from build123d import *

# Parameters (mm, degrees)
F0_R          = 10
F1_DEPTH      = 45
F1_DEPTH_BACK = 95
F0_R_2        = 15
F2_DEPTH      = 65
F4_START      = 7.5
F4_DEPTH      = 17.5
F6_DEPTH      = 30
F7_R          = 2
F8_DEPTH      = 25
F9_R          = 2
F10_DEPTH     = 25
F11_R         = 2
F12_DEPTH     = 25
F13_R         = 2
F14_DEPTH     = 25
F16_D         = 5
F16_DEPTH     = 20
F16_TIP       = 1.5021515476
F17_R         = 11.65
F18_DEPTH     = 1


with BuildPart() as f1:
    # F0 (on Front) → F1 (new body, two sides)
    with BuildSketch(Plane.XZ) as f1_sk:
        Circle(F0_R)
    extrude(amount=F1_DEPTH)
    extrude(f1_sk.sketch, amount=-F1_DEPTH_BACK)

    # F0 (on Front) → F2 (join)
    with BuildSketch(Plane.XZ):
        Circle(F0_R_2)
        Circle(F0_R, mode=Mode.SUBTRACT)
    extrude(amount=-F2_DEPTH)

    # F3 (on Top) → F4 (cut)
    with BuildSketch(Plane.XY.offset(F4_START)):
        with BuildLine():
            ThreePointArc((2.5, 75), (0, 77.5), (-2.5, 75))
            Line((-2.5, 75), (2.5, 75))
        make_face()
        with BuildLine():
            ThreePointArc((0, 72.5), (-1.767766953, 73.232233047), (-2.5, 75))
            Line((-2.5, 75), (-2.5, 70))
            ThreePointArc((-2.5, 70), (-1.767766953, 71.767766953), (0, 72.5))
        make_face()
        with BuildLine():
            Line((2.5, 75), (-2.5, 75))
            ThreePointArc((-2.5, 75), (-1.767766953, 73.232233047), (0, 72.5))
            ThreePointArc((0, 72.5), (1.767766953, 73.232233047), (2.5, 75))
        make_face()
        with BuildLine():
            Line((2.5, 70), (2.5, 75))
            ThreePointArc((2.5, 75), (1.767766953, 73.232233047), (0, 72.5))
            ThreePointArc((0, 72.5), (1.767766953, 71.767766953), (2.5, 70))
        make_face()
        with BuildLine():
            ThreePointArc((0, 72.5), (-1.767766953, 71.767766953), (-2.5, 70))
            Line((-2.5, 70), (2.5, 70))
            ThreePointArc((2.5, 70), (1.767766953, 71.767766953), (0, 72.5))
        make_face()
        with BuildLine():
            Line((2.5, 70), (-2.5, 70))
            ThreePointArc((-2.5, 70), (0, 67.5), (2.5, 70))
        make_face()
    extrude(amount=F4_DEPTH, mode=Mode.SUBTRACT)

    # F5 (on face) → F6 (cut)
    with BuildSketch(Plane.XZ.offset(45)):
        with BuildLine():
            Line((2, 8), (2, 9.7979589711))
            ThreePointArc((2, 9.7979589711), (0, 10), (-2, 9.7979589711))
            Line((-2, 9.7979589711), (-2, 8))
            Line((-2, 8), (2, 8))
        make_face()
        with BuildLine():
            ThreePointArc((9.7979589711, -2), (9.9493615301, -1.0050896201), (10, 0))
            ThreePointArc((10, 0), (9.9493615301, 1.0050896201), (9.7979589711, 2))
            Line((9.7979589711, 2), (8, 2))
            Line((8, 2), (8, -2))
            Line((8, -2), (9.7979589711, -2))
        make_face()
        with BuildLine():
            ThreePointArc((-2, -9.7979589711), (0, -10), (2, -9.7979589711))
            Line((2, -9.7979589711), (2, -8))
            Line((2, -8), (-2, -8))
            Line((-2, -8), (-2, -9.7979589711))
        make_face()
        with BuildLine():
            Line((-8, 2), (-9.7979589711, 2))
            ThreePointArc((-9.7979589711, 2), (-10, 0), (-9.7979589711, -2))
            Line((-9.7979589711, -2), (-8, -2))
            Line((-8, -2), (-8, 2))
        make_face()
    extrude(amount=-F6_DEPTH, mode=Mode.SUBTRACT)

    # F7 (on face) → F8 (cut)
    with BuildSketch(Plane.XY.offset(8)):
        with Locations((0, -15)):
            Circle(F7_R)
    extrude(amount=F8_DEPTH, mode=Mode.SUBTRACT)

    # F9 (on face) → F10 (cut)
    with BuildSketch(Plane.YZ.offset(8)):
        with Locations((-15, 0)):
            Circle(F9_R)
    extrude(amount=F10_DEPTH, mode=Mode.SUBTRACT)

    # F11 (on face) → F12 (cut)
    with BuildSketch(Plane(origin=(0, 0, -8), x_dir=(1, 0, 0), z_dir=(0, 0, -1))):
        with Locations((0, 15)):
            Circle(F11_R)
    extrude(amount=F12_DEPTH, mode=Mode.SUBTRACT)

    # F13 (on face) → F14 (cut)
    with BuildSketch(Plane(origin=(-8, 0, 0), x_dir=(0, -1, 0), z_dir=(-1, 0, 0))):
        with Locations((15, 0)):
            Circle(F13_R)
    extrude(amount=F14_DEPTH, mode=Mode.SUBTRACT)

    # F16
    with Locations(Plane.XZ.offset(45)):
        with Locations((0, 0)):
            Hole(F16_D / 2, depth=F16_DEPTH)
            with Locations((0, 0, -(F16_DEPTH + F16_TIP / 2))):  # 118° drill point
                Cone(0, F16_D / 2, F16_TIP, mode=Mode.SUBTRACT)

    # F17 (on face) → F18 (join)
    with BuildSketch(Plane.XZ):
        Circle(F17_R)
    extrude(amount=F18_DEPTH)


solid = f1.part
Geometry check sheet. Reference: the model listing, model coordinates, mm. A direction names the side the tool comes from. Round coordinates to 2 decimals unless told otherwise and drop trailing zeros. Write each loop counter-clockwise with the first axis right and the second up, starting at its lowest first coordinate (ties: lowest second). Pieces come first, ordered by that corner, then holes. Notation, with made-up numbers: (-10, 26) -> (-6, 26) arc R16 ccw to (-6, 40) -> close; hole circle Ø6 at (-36.5, 78.25). An arc over 180 degrees is marked (long way). One line per item, written item: value. Start each with the question number.
(1) Scan lines: line 1 (X direction, y = -40, z = 0); line 2 (Y direction, x = 8.5, z = 5.75). Record each from-to range of solid material in increasing order. Write a range as [from, to].
(2) Cross-section at B-B, the plane x = -6. Record the cut outline in (y, z), and give its area (3 significant figures).
(3) Cross-section at D-D, the plane z = 13. Record the cut outline in (x, y), and give its area (3 significant figures).
(4) Access from +Z, -Z, +X, -X, +Y, -Y to the whole of each face (thin tool, end or side, straight path). Record for faces 4 (the cylindrical face through (0.54, -34.86, -2.44)), 5 (the flat face through (0, 73, 7.5)), 6 (the cylindrical face through (-2.17, 79.79, -9.76)), 7 (the flat face through (0, -29, 8)), 8 (the flat face through (0, -29, -8)).
(5) Cross-section at C-C, the plane y = 80. Record the cut outline in (x, z).
(6) Cross-section at A-A, the plane y = -28. Record the cut outline in (x, z).
(7) Draft check along X on faces 1 (the flat face through (0, 95, 0)), 2 (the cylindrical face through (-2.53, -0.49, -11.37)), 3 (the cylindrical face through (-0.1, 67.5, 8.7)). Enter one of: +X half, -X half, draft (parallel to the pull), parting line (faces both ways), or undercut.
(8) Go/stop test with flat-tipped pins: pin 1 Ø3 at (y, z) = (65.5, -9) entering from +X; pin 2 Ø0.9 at (y, z) = (-26.5, 9) entering from -X; pin 3 Ø2 at (x, z) = (-3.5, 10.5) entering from -Y. Record where each tip stops, or that it passes through.
Answer:
1. line 1: [-8, -2.5], [2.5, 8]
1. line 2: [-1, 65]
2. outline: (-45, -8) -> (-1, -8) -> (-1, -9.99) -> (0, -9.99) -> (0, -13.75) -> (65, -13.75) -> (65, -8) -> (95, -8) -> (95, 8) -> (65, 8) -> (65, 13.75) -> (0, 13.75) -> (0, 9.99) -> (-1, 9.99) -> (-1, 8) -> (-45, 8) -> close
2. area: 2,990 mm²
3. outline: (-7.48, 0) -> (7.48, 0) -> (7.48, 65) -> (-7.48, 65) -> close
3. area: 973 mm²
4. face 4: -Y
4. face 5: +Z
4. face 6: +Y
4. face 7: +Z, -Y
4. face 8: -Z, -Y
5. outline: circle Ø20 at (0, 0)
6. outline: (-9.8, -2) arc R10 ccw to (-2, -9.8) -> (-2, -8) -> (2, -8) -> (2, -9.8) arc R10 ccw to (9.8, -2) -> (8, -2) -> (8, 2) -> (9.8, 2) arc R10 ccw to (2, 9.8) -> (2, 8) -> (-2, 8) -> (-2, 9.8) arc R10 ccw to (-9.8, 2) -> (-8, 2) -> (-8, -2) -> close; hole circle Ø5 at (0, 0)
7. face 1: draft
7. face 2: parting line
7. face 3: undercut
8. pin 1: x = 12.94
8. pin 2: x = -5.19
8. pin 3: y = -1
